```python
from build123d import *

# Parameters (mm, degrees)
SKETCH_1_W          = 15
SKETCH_1_H          = 10
SKETCH_1_W_2        = 13
SKETCH_1_H_2        = 8
EXTRUDE_1_DEPTH     = 40
CUT_EXTRUDE_1_REACH = 45.875
SKETCH_2_R          = 1.6
SKETCH_2_R_2        = 2.15


with BuildPart() as part:
    # ｽｹｯﾁ1 → 押し出し-薄板1 (new body)
    with BuildSketch(Plane.XY):
        with Locations((7.5, 5)):
            Rectangle(SKETCH_1_W, SKETCH_1_H)
        with Locations((7.5, 5)):
            Rectangle(SKETCH_1_W_2, SKETCH_1_H_2, mode=Mode.SUBTRACT)
    extrude(amount=EXTRUDE_1_DEPTH)

    # ｶｯﾄ - 押し出し1: up to this face of the body (flat: up to its plane)
    cut_extrude_1_end = Plane(part.part.faces().sort_by_distance((0, 5, 20))[0])
    # ｽｹｯﾁ2 → ｶｯﾄ - 押し出し1 (cut, up to the picked face)
    with BuildSketch(Plane(origin=(15, 0, 0), x_dir=(0, 0, -1), z_dir=(1, 0, 0)), mode=Mode.PRIVATE) as cut_extrude_1_sk1:
        with Locations((-5, 5)):
            Circle(SKETCH_2_R)
    cut_extrude_1_tool1 = split(extrude(cut_extrude_1_sk1.sketch, amount=-CUT_EXTRUDE_1_REACH, mode=Mode.PRIVATE), bisect_by=cut_extrude_1_end, keep=Keep.BOTH, mode=Mode.PRIVATE)
    # ｽｹｯﾁ2 → ｶｯﾄ - 押し出し1 (cut, up to the picked face)
    with BuildSketch(Plane(origin=(15, 0, 0), x_dir=(0, 0, -1), z_dir=(1, 0, 0)), mode=Mode.PRIVATE) as cut_extrude_1_sk2:
        with Locations((-15, 5)):
            Circle(SKETCH_2_R)
    cut_extrude_1_tool2 = split(extrude(cut_extrude_1_sk2.sketch, amount=-CUT_EXTRUDE_1_REACH, mode=Mode.PRIVATE), bisect_by=cut_extrude_1_end, keep=Keep.BOTH, mode=Mode.PRIVATE)
    # ｽｹｯﾁ2 → ｶｯﾄ - 押し出し1 (cut, up to the picked face)
    with BuildSketch(Plane(origin=(15, 0, 0), x_dir=(0, 0, -1), z_dir=(1, 0, 0)), mode=Mode.PRIVATE) as cut_extrude_1_sk3:
        with Locations((-35, 5)):
            Circle(SKETCH_2_R_2)
    cut_extrude_1_tool3 = split(extrude(cut_extrude_1_sk3.sketch, amount=-CUT_EXTRUDE_1_REACH, mode=Mode.PRIVATE), bisect_by=cut_extrude_1_end, keep=Keep.BOTH, mode=Mode.PRIVATE)
    add(cut_extrude_1_tool1.solids().sort_by(Axis((15, 5, 5), (-1, 0, 0)))[0], mode=Mode.SUBTRACT)
    add(cut_extrude_1_tool2.solids().sort_by(Axis((15, 5, 15), (-1, 0, 0)))[0], mode=Mode.SUBTRACT)
    add(cut_extrude_1_tool3.solids().sort_by(Axis((15, 5, 35), (-1, 0, 0)))[0], mode=Mode.SUBTRACT)


solid = part.part
```
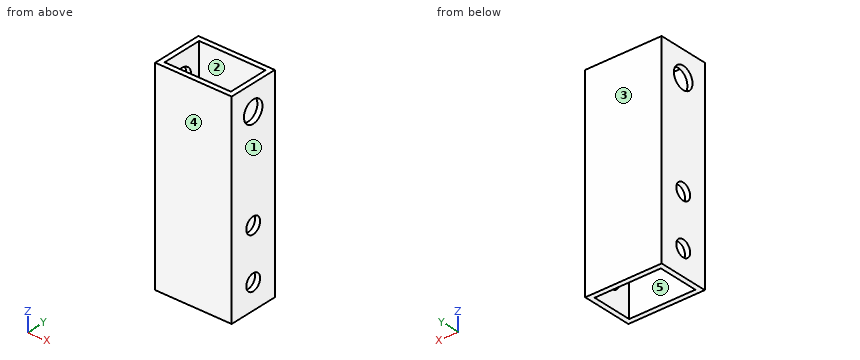
CAD build for the part. Positions are in the model's coordinates, mm. Face numbers are marked on the shaded views. A direction names the side the tool comes from. Round coordinates to 2 decimals unless told otherwise and drop trailing zeros. Loops run counter-clockwise (first coordinate to the right, second up) from the corner with the lowest first, then second, coordinate; pieces in that order, holes last. Notation, with made-up numbers: M 71.5,66 L 128.5,66 A15 ccw 128.5,83 Z; hole C -4.75,21 d11. An arc over 180 degrees is marked long. Return JSON: item names as keys, results as strings. Group by question number.
(1) Drop a flat-ended pin along its axis: P1, Ø4, axis at x = 7.5, y = 9, coming from the -Z side. Give the stop position or say it passes through.
(2) Wall check: probe 1 along X at (y, z) = (1.25, 31); probe 2 along Y at (x, z) = (14.35, 35); probe 3 along Y at (x, z) = (13.5, 18.5). Give the ranges that are in metal, low to high. Write a range as [from, to].
(3) Saw through at A-A, the plane z = 35. List the corners of the cut face in (x, y), and give its area (3 significant figures).
(4) Tool access for the marked faces 4 and 5: list every direction of +Z, -Z, +X, -X, +Y, -Y with a clear straight run to the whole face (end or side of a thin tool).
(5) Saw through at D-D, the plane z = 31. List the corners of the cut face in (x, y).
(6) Saw through at C-C, the plane x = 6.75. List the corners of the cut face in (y, z), and give its area (3 significant figures).
(7) Saw through at B-B, the plane y = 2.25. List the corners of the cut face in (x, z).
(8) Mould opens along X. For the marked faces 1, 2 and 3 say: +X half, -X half, draft (parallel to the pull), parting line (faces both ways), or undercut.
Answer list:
{
 "1": {"P1": "z = 0"},
 "2": {"probe 1": "[0, 1], [14, 15]", "probe 2": "[0, 2.85], [7.15, 10]", "probe 3": "[0, 1], [9, 10]"},
 "3": {"outline": "M 0,0 L 15,0 L 15,2.85 L 14,2.85 L 14,1 L 1,1 L 1,2.85 L 0,2.85 Z; M 0,7.15 L 1,7.15 L 1,9 L 14,9 L 14,7.15 L 15,7.15 L 15,10 L 0,10 Z", "area": "37.4 mm2"},
 "4": {"face 4": "+Z, -Z, +X, -X, -Y", "face 5": "+Z, -Z"},
 "5": {"outline": "M 0,0 L 15,0 L 15,10 L 0,10 Z; hole M 1,1 L 14,1 L 14,9 L 1,9 Z"},
 "6": {"outline": "M 0,0 L 1,0 L 1,40 L 0,40 Z; M 9,0 L 10,0 L 10,40 L 9,40 Z", "area": "80.0 mm2"},
 "7": {"outline": "M 0,0 L 1,0 L 1,40 L 0,40 Z; M 14,0 L 15,0 L 15,40 L 14,40 Z"},
 "8": {"face 1": "+X half", "face 2": "undercut", "face 3": "draft"}
}
